```python
from build123d import *

# Parameters (mm, degrees)
F0_R     = 2.5
F1_DEPTH = 5
F2_R     = 2
F3_DEPTH = 4
F5_DEPTH = 3
F6_W     = 2
F6_H     = 1.83
F7_DEPTH = 3


with BuildPart() as f1:
    # F0 (on Top) → F1 (new body)
    with BuildSketch(Plane.XY):
        Circle(F0_R)
    extrude(amount=F1_DEPTH)

    # F2 (on face) → F3 (cut)
    with BuildSketch(Plane.XY.offset(5)):
        Circle(F2_R)
    extrude(amount=-F3_DEPTH, mode=Mode.SUBTRACT)

    # F4 (on face) → F5 (cut)
    with BuildSketch(Plane.XY.offset(5)):
        with BuildLine():
            ThreePointArc((-1, -2.2912878475), (0, -2.5), (1, -2.2912878475))
            Line((1, -2.2912878475), (1, -1.7320508076))
            ThreePointArc((1, -1.7320508076), (0, -2), (-1, -1.7320508076))
            Line((-1, -1.7320508076), (-1, -2.2912878475))
        make_face()
    extrude(amount=-F5_DEPTH, mode=Mode.SUBTRACT)

    # F6 (on face) → F7 (cut)
    with BuildSketch(Plane.XY.offset(5)):
        with Locations((0, 2)):
            Rectangle(F6_W, F6_H)
    extrude(amount=-F7_DEPTH, mode=Mode.SUBTRACT)


solid = f1.part
```
Geometry: final body of the model. Coordinates: model frame, mm. A direction names the side the tool comes from. Coordinates: 2 decimals unless noted, no trailing zeros. Order: outer loops, then holes, each group sorted by start corner. A loop starts at its lowest first (then second) coordinate and runs counter-clockwise, first axis right, second up. Notation, with made-up numbers: (-5, 46) - (30, 46) arc R24 cw to (30, 80) - close; hole circle Ø8 at (81, -11.75). An arc over 180 degrees is marked (long way). Write each question's results on one line, items separated by ' | '.
1) Set-up query: faces 1 (the flat face through (-2.3, 0, 5)), 2 (the cylindrical face through (-1.474, 1.352, 3.028)). Return all of +Z, -Z, +X, -X, +Y, -Y with unobstructed straight access to the full face (end or side cutting, diameter ignored); none if empty.
Results list:
face 1: +Z, +X, -X, +Y, -Y | face 2: +Z
2) Section B-B, the plane y = 0. Return loops of the section in (x, z), plus the area to 3 significant figures.
Results list:
outline: (-2.5, 0) - (2.5, 0) - (2.5, 5) - (2, 5) - (2, 1) - (-2, 1) - (-2, 5) - (-2.5, 5) - close | area: 9.00 mm^2
3) Line query: line 1 (X direction, y = 0, z = 3.85); line 2 (X direction, y = 0.1, z = 0.5); line 3 (Z direction, x = -0.7, y = -1.3). Output: solid intervals per line, ascending. Write a range as from..to.
Results list:
line 1: -2.5..-2, 2..2.5 | line 2: -2.5..2.5 | line 3: 0..1
4) Section A-A, the plane z = 3.85. Return loops of the section in (x, y).
Results list:
outline: (-1, -2.29) - (-1, -1.73) arc R2 cw to (-1, 1.73) - (-1, 2.29) arc R2.5 ccw to start; (1, -2.29) arc R2.5 ccw to (1, 2.29) - (1, 1.73) arc R2 cw to (1, -1.73) - close
5) Pin query (flat end, axial travel): pin 1 (3 mm diameter, centred on x = 0, y = -1, fed in from +Z); pin 2 (1.5 mm diameter, centred on x = 1.5, z = 1, fed in from -Y); pin 3 (0.6 mm diameter, centred on y = -2, z = 4, fed in from -X); pin 4 (1 mm diameter, centred on x = 1, z = 4.5, fed in from +Y). Return the tip coordinate at first contact, or that it passes through.
Results list:
pin 1: z = 5 | pin 2: y = -2.38 | pin 3: x = -1.83 | pin 4: y = 2.29
6) Pull-direction query (Y, two-part tool) for faces 3 (the flat face through (2.2, -0.2, 5)), 4 (the cylindrical face through (2.31, -0.96, 2.46)), 5 (the flat face through (0, 0, 1)); classes: pulls with the +Y half, pulls with the -Y half, needs draft (parallel to the pull), parting line crosses it, or undercut.
Results list:
face 3: needs draft | face 4: parting line crosses it | face 5: undercut
7) Section C-C, the plane x = 0. Return loops of the section in (y, z).
Results list:
outline: (-2.5, 0) - (2.5, 0) - (2.5, 2) - (2, 2) - (2, 1) - (-2, 1) - (-2, 2) - (-2.5, 2) - close
